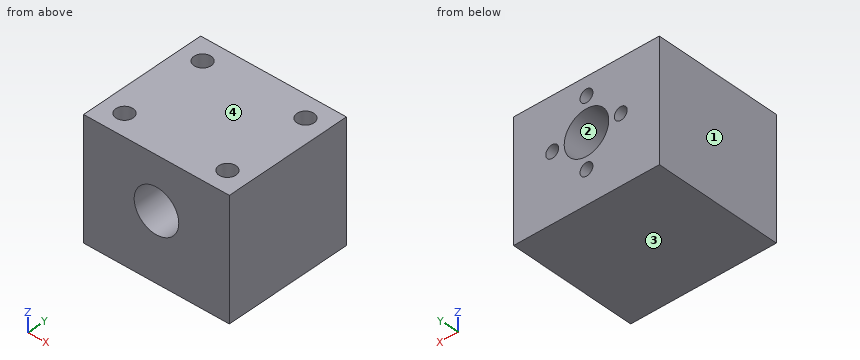
```python
from build123d import *

# Parameters (mm, degrees)
SKETCH_1_W          = 34
SKETCH_1_H          = 30
EXTRUDE_1_DEPTH     = 28
SKETCH_2_R          = 2
CUT_EXTRUDE_1_DEPTH = 7
SKETCH_3_R          = 5.2
CUT_EXTRUDE_3_DEPTH = 31
SKETCH_5_R          = 1.5
CUT_EXTRUDE_4_DEPTH = 7


with BuildPart() as part:
    # 草图1 → 凸台-拉伸1 (new body)
    with BuildSketch(Plane.XY):
        with Locations((0.688013078, -5.139852888)):
            Rectangle(SKETCH_1_W, SKETCH_1_H)
    extrude(amount=-EXTRUDE_1_DEPTH)

    # 草图2 → 切除-拉伸1 (cut)
    with BuildSketch(Plane.XY):
        with Locations((-11.311986922, 4.86014711)):
            Circle(SKETCH_2_R)
        with Locations((12.688013078, 4.86014711)):
            Circle(SKETCH_2_R)
        with Locations((12.688013078, -15.13985289)):
            Circle(SKETCH_2_R)
        with Locations((-11.311986922, -15.13985289)):
            Circle(SKETCH_2_R)
    extrude(amount=-CUT_EXTRUDE_1_DEPTH, mode=Mode.SUBTRACT)

    # 草图3 → 切除-拉伸3 (cut, through all)
    with BuildSketch(Plane(origin=(0, 9.860147112, 0), x_dir=(1, 0, 0), z_dir=(0, 1, 0))):
        with Locations((0.688013078, 12.2)):
            Circle(SKETCH_3_R)
    extrude(amount=-CUT_EXTRUDE_3_DEPTH, mode=Mode.SUBTRACT)

    # 草图5 → 切除-拉伸4 (cut)
    with BuildSketch(Plane(origin=(0, 9.860147112, 0), x_dir=(1, 0, 0), z_dir=(0, 1, 0))):
        with Locations((0.688013078, 4.2)):
            Circle(SKETCH_5_R)
        with Locations((8.688013078, 12.2)):
            Circle(SKETCH_5_R)
        with Locations((0.688013078, 20.2)):
            Circle(SKETCH_5_R)
        with Locations((-7.311986922, 12.2)):
            Circle(SKETCH_5_R)
    extrude(amount=-CUT_EXTRUDE_4_DEPTH, mode=Mode.SUBTRACT)


solid = part.part
```
Can you work these out from the model? Positions are in its coordinate system, mm. Face numbers are marked on the shaded views. Coordinates: 2 decimals unless noted, no trailing zeros. Loops run counter-clockwise (first coordinate to the right, second up) from the corner with the lowest first, then second, coordinate; pieces in that order, holes last.
Item 1: Please list where these lines run through material, in increasing order: L1, parallel to X at y = 7, z = -12.2; L2, parallel to X at y = 7.5, z = -20.2; L3, parallel to X at y = -17, z = -16.
Answers below:
L1: x = -16.31 to -8.81, -5.81 to -4.51, 5.89 to 7.19, 10.19 to 17.69
L2: x = -16.31 to -0.81, 2.19 to 17.69
L3: x = -16.31 to -2.86, 4.24 to 17.69
Item 2: Suppose I cut it at C-C (z = -20.2). Please give me the cut outline in (x, y).
Answers below:
outline: (-16.31, -20.14) - (17.69, -20.14) - (17.69, 9.86) - (2.19, 9.86) - (2.19, 2.86) - (-0.81, 2.86) - (-0.81, 9.86) - (-16.31, 9.86) - close
Item 3: I'm going to push flat-ended pins straight in: pin 1 (9.5 mm diameter, centred on x = 0.69, z = -12.2, fed in from +Y); pin 2 (3.5 mm diameter, centred on x = 12.69, y = -15.14, fed in from +Z); pin 3 (0.9 mm diameter, centred on x = -8, z = -12.5, fed in from +Y). Where does each tip first touch, or does it pass through?
Answers below:
pin 1: passes through
pin 2: stops at z = -7
pin 3: stops at y = 2.86
Item 4: Suppose I cut it at A-A (z = -12.2). Please give me the cut outline in (x, y).
Answers below:
outline: (-16.31, -20.14) - (-4.51, -20.14) - (-4.51, 9.86) - (-5.81, 9.86) - (-5.81, 2.86) - (-8.81, 2.86) - (-8.81, 9.86) - (-16.31, 9.86) - close; (5.89, -20.14) - (17.69, -20.14) - (17.69, 9.86) - (10.19, 9.86) - (10.19, 2.86) - (7.19, 2.86) - (7.19, 9.86) - (5.89, 9.86) - close
Item 5: Suppose I cut it at D-D (y = 5.75). Please give me the cut outline in (x, z).
Answers below:
outline: (-16.31, -28) - (17.69, -28) - (17.69, 0) - (14.48, 0) - (14.48, -7) - (10.9, -7) - (10.9, 0) - (-9.52, 0) - (-9.52, -7) - (-13.1, -7) - (-13.1, 0) - (-16.31, 0) - close; hole circle Ø3 at (-7.31, -12.2); hole circle Ø10.4 at (0.69, -12.2); hole circle Ø3 at (0.69, -20.2); hole circle Ø3 at (0.69, -4.2); hole circle Ø3 at (8.69, -12.2)
Item 6: Suppose I cut it at B-B (y = -8.75). Please give me the cut outline in (x, z).
Answers below:
outline: (-16.31, -28) - (17.69, -28) - (17.69, 0) - (-16.31, 0) - close; hole circle Ø10.4 at (0.69, -12.2)
Item 7: If we mould it in two halves opening along Z, with no side actions, what happens to the marked faces 1, 2, 3 and 4? For each: released by +Z, released by -Z, zero draft, split by the parting line, or undercut.
Answers below:
face 1: zero draft
face 2: undercut
face 3: released by -Z
face 4: released by +Z
